```python
from build123d import *

# Parameters (mm, degrees)
SKETCH1_W                   = 3.2
SKETCH1_H                   = 10.1
BOSS_EXTRUDE1_DEPTH         = 3
SENSOR_MOUNTING_HOLES_REACH = 85.637
SKETCH2_R                   = 1.6
SKETCH2_R_2                 = 1.5
SKETCH2_R_3                 = 3.1
SKETCH2_W                   = 9.5
SKETCH2_H                   = 8
SKETCH2_W_2                 = 29.5
SKETCH2_H_2                 = 8.4
SKETCH2_W_3                 = 11.5
SKETCH2_H_3                 = 13
SKETCH2_W_4                 = 12
SKETCH2_H_4                 = 11


with BuildPart() as part:
    # Sketch1 → Boss-Extrude1 (new body)
    with BuildSketch(Plane.XY):
        with BuildLine():
            Line((-58.19, 60), (58.19, 60))
            Line((58.19, 60), (58.19, 3))
            Line((58.19, 3), (11.618950039, 3))
            ThreePointArc((11.618950039, 3), (0, 12), (-11.618950039, 3))
            Line((-11.618950039, 3), (-58.19, 3))
            Line((-58.19, 3), (-58.19, 60))
        make_face()
        with Locations((-52.69, 15)):
            Rectangle(SKETCH1_W, SKETCH1_H, mode=Mode.SUBTRACT)
        with Locations((-52.69, 48)):
            Rectangle(SKETCH1_W, SKETCH1_H, mode=Mode.SUBTRACT)
        with Locations((52.69, 15)):
            Rectangle(SKETCH1_W, SKETCH1_H, mode=Mode.SUBTRACT)
        with Locations((52.69, 48)):
            Rectangle(SKETCH1_W, SKETCH1_H, mode=Mode.SUBTRACT)
    extrude(amount=-BOSS_EXTRUDE1_DEPTH)

    # Sketch2 (on Front Plane) → sensor mounting holes (cut, up to next)
    with BuildSketch(Plane.XY, mode=Mode.PRIVATE) as sensor_mounting_holes_sk1:
        with Locations((-18, 44)):
            Circle(SKETCH2_R)
    sensor_mounting_holes_tool1 = extrude(sensor_mounting_holes_sk1.sketch, amount=-SENSOR_MOUNTING_HOLES_REACH, mode=Mode.PRIVATE) & part.part
    # Sketch2 (on Front Plane) → sensor mounting holes (cut, up to next)
    with BuildSketch(Plane.XY, mode=Mode.PRIVATE) as sensor_mounting_holes_sk2:
        with Locations((18, 44)):
            Circle(SKETCH2_R)
    sensor_mounting_holes_tool2 = extrude(sensor_mounting_holes_sk2.sketch, amount=-SENSOR_MOUNTING_HOLES_REACH, mode=Mode.PRIVATE) & part.part
    # Sketch2 (on Front Plane) → sensor mounting holes (cut, up to next)
    with BuildSketch(Plane.XY, mode=Mode.PRIVATE) as sensor_mounting_holes_sk3:
        with Locations((-22.118932188, 29.071067812)):
            Circle(SKETCH2_R_2)
    sensor_mounting_holes_tool3 = extrude(sensor_mounting_holes_sk3.sketch, amount=-SENSOR_MOUNTING_HOLES_REACH, mode=Mode.PRIVATE) & part.part
    # Sketch2 (on Front Plane) → sensor mounting holes (cut, up to next)
    with BuildSketch(Plane.XY, mode=Mode.PRIVATE) as sensor_mounting_holes_sk4:
        with Locations((-36.261067812, 29.071067812)):
            Circle(SKETCH2_R_2)
    sensor_mounting_holes_tool4 = extrude(sensor_mounting_holes_sk4.sketch, amount=-SENSOR_MOUNTING_HOLES_REACH, mode=Mode.PRIVATE) & part.part
    # Sketch2 (on Front Plane) → sensor mounting holes (cut, up to next)
    with BuildSketch(Plane.XY, mode=Mode.PRIVATE) as sensor_mounting_holes_sk5:
        with Locations((-36.261067812, 14.928932188)):
            Circle(SKETCH2_R_2)
    sensor_mounting_holes_tool5 = extrude(sensor_mounting_holes_sk5.sketch, amount=-SENSOR_MOUNTING_HOLES_REACH, mode=Mode.PRIVATE) & part.part
    # Sketch2 (on Front Plane) → sensor mounting holes (cut, up to next)
    with BuildSketch(Plane.XY, mode=Mode.PRIVATE) as sensor_mounting_holes_sk6:
        with Locations((-22.118932188, 14.928932188)):
            Circle(SKETCH2_R_2)
    sensor_mounting_holes_tool6 = extrude(sensor_mounting_holes_sk6.sketch, amount=-SENSOR_MOUNTING_HOLES_REACH, mode=Mode.PRIVATE) & part.part
    # Sketch2 (on Front Plane) → sensor mounting holes (cut, up to next)
    with BuildSketch(Plane.XY, mode=Mode.PRIVATE) as sensor_mounting_holes_sk7:
        with Locations((-29.19, 22)):
            Circle(SKETCH2_R_2)
    sensor_mounting_holes_tool7 = extrude(sensor_mounting_holes_sk7.sketch, amount=-SENSOR_MOUNTING_HOLES_REACH, mode=Mode.PRIVATE) & part.part
    # Sketch2 (on Front Plane) → sensor mounting holes (cut, up to next)
    with BuildSketch(Plane.XY, mode=Mode.PRIVATE) as sensor_mounting_holes_sk8:
        with Locations((30.240588995, 13.245945843)):
            Circle(SKETCH2_R_3)
    sensor_mounting_holes_tool8 = extrude(sensor_mounting_holes_sk8.sketch, amount=-SENSOR_MOUNTING_HOLES_REACH, mode=Mode.PRIVATE) & part.part
    # Sketch2 (on Front Plane) → sensor mounting holes (cut, up to next)
    with BuildSketch(Plane.XY, mode=Mode.PRIVATE) as sensor_mounting_holes_sk9:
        with Locations((16.44, 27)):
            Rectangle(SKETCH2_W, SKETCH2_H)
    sensor_mounting_holes_tool9 = extrude(sensor_mounting_holes_sk9.sketch, amount=-SENSOR_MOUNTING_HOLES_REACH, mode=Mode.PRIVATE) & part.part
    # Sketch2 (on Front Plane) → sensor mounting holes (cut, up to next)
    with BuildSketch(Plane.XY, mode=Mode.PRIVATE) as sensor_mounting_holes_sk10:
        with Locations((0, 44)):
            Rectangle(SKETCH2_W_2, SKETCH2_H_2)
    sensor_mounting_holes_tool10 = extrude(sensor_mounting_holes_sk10.sketch, amount=-SENSOR_MOUNTING_HOLES_REACH, mode=Mode.PRIVATE) & part.part
    # Sketch2 (on Front Plane) → sensor mounting holes (cut, up to next)
    with BuildSketch(Plane.XY, mode=Mode.PRIVATE) as sensor_mounting_holes_sk11:
        Polygon((24.912246381, 42.955051143), (29.112246381, 42.955051143), (29.112246381, 51.455051143), (32.612246381, 51.455051143), (32.612246381, 25.155051143), (29.112246381, 25.155051143), (29.112246381, 34.655051143), (24.912246381, 34.655051143), align=None)
    sensor_mounting_holes_tool11 = extrude(sensor_mounting_holes_sk11.sketch, amount=-SENSOR_MOUNTING_HOLES_REACH, mode=Mode.PRIVATE) & part.part
    # Sketch2 (on Front Plane) → sensor mounting holes (cut, up to next)
    with BuildSketch(Plane.XY, mode=Mode.PRIVATE) as sensor_mounting_holes_sk12:
        with Locations((41.090588995, 19.745945843)):
            Rectangle(SKETCH2_W_3, SKETCH2_H_3)
    sensor_mounting_holes_tool12 = extrude(sensor_mounting_holes_sk12.sketch, amount=-SENSOR_MOUNTING_HOLES_REACH, mode=Mode.PRIVATE) & part.part
    # Sketch2 (on Front Plane) → sensor mounting holes (cut, up to next)
    with BuildSketch(Plane.XY, mode=Mode.PRIVATE) as sensor_mounting_holes_sk13:
        with Locations((40.362246381, 49.88070744)):
            Rectangle(SKETCH2_W_4, SKETCH2_H_4)
    sensor_mounting_holes_tool13 = extrude(sensor_mounting_holes_sk13.sketch, amount=-SENSOR_MOUNTING_HOLES_REACH, mode=Mode.PRIVATE) & part.part
    add(sensor_mounting_holes_tool1.solids().sort_by_distance((-18, 44, 0))[0], mode=Mode.SUBTRACT)
    add(sensor_mounting_holes_tool2.solids().sort_by_distance((18, 44, 0))[0], mode=Mode.SUBTRACT)
    add(sensor_mounting_holes_tool3.solids().sort_by_distance((-22.118932, 29.071068, 0))[0], mode=Mode.SUBTRACT)
    add(sensor_mounting_holes_tool4.solids().sort_by_distance((-36.261068, 29.071068, 0))[0], mode=Mode.SUBTRACT)
    add(sensor_mounting_holes_tool5.solids().sort_by_distance((-36.261068, 14.928932, 0))[0], mode=Mode.SUBTRACT)
    add(sensor_mounting_holes_tool6.solids().sort_by_distance((-22.118932, 14.928932, 0))[0], mode=Mode.SUBTRACT)
    add(sensor_mounting_holes_tool7.solids().sort_by_distance((-29.19, 22, 0))[0], mode=Mode.SUBTRACT)
    add(sensor_mounting_holes_tool8.solids().sort_by_distance((30.240589, 13.245946, 0))[0], mode=Mode.SUBTRACT)
    add(sensor_mounting_holes_tool9.solids().sort_by_distance((16.44, 27, 0))[0], mode=Mode.SUBTRACT)
    add(sensor_mounting_holes_tool10.solids().sort_by_distance((0, 44, 0))[0], mode=Mode.SUBTRACT)
    add(sensor_mounting_holes_tool11.solids().sort_by_distance((29.804717, 38.442393, 0))[0], mode=Mode.SUBTRACT)
    add(sensor_mounting_holes_tool12.solids().sort_by_distance((41.090589, 19.745946, 0))[0], mode=Mode.SUBTRACT)
    add(sensor_mounting_holes_tool13.solids().sort_by_distance((40.362246, 49.880707, 0))[0], mode=Mode.SUBTRACT)


solid = part.part
```
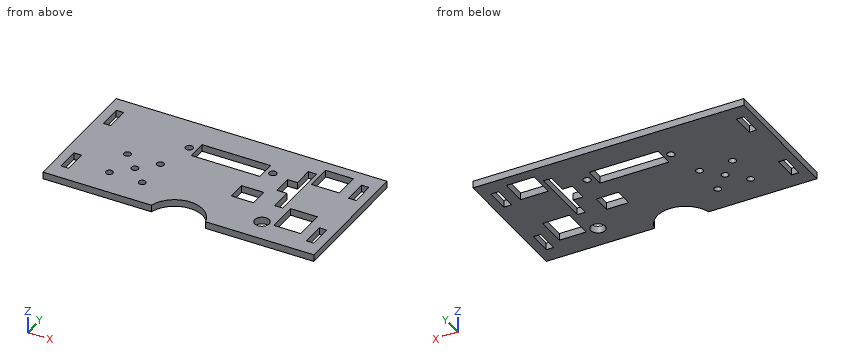
CAD build for the part. Positions are in the model's coordinates, mm. Round coordinates to 2 decimals unless told otherwise and drop trailing zeros. Write each loop counter-clockwise with the first axis right and the second up, starting at its lowest first coordinate (ties: lowest second). Pieces come first, ordered by that corner, then holes. Notation, with made-up numbers: (49.5, 39) -> (77.5, 39) arc R25 ccw to (77.5, 60) -> close; hole circle Ø10 at (24.5, -31.75). An arc over 180 degrees is marked (long way). Answer in a Markdown table with one row per item. Add a question column.
Item 1: Drill centre lines: line 1 (Y direction, x = 43, z = -0.8); line 2 (X direction, y = 41.5, z = -1.9); line 3 (X direction, y = 52, z = -1.6). Where is each one in solid material? Low to high. Write a range as from..to.
Item 2: Saw through at B-B, the plane y = 6. Write the cut outline in (x, z), then the cut area to 3 significant figures.
Item 3: Saw through at C-C, the plane z = -1.85. Count the separate pieces of the cut face and the enclosed holes in it, then the cut area to 3 significant figures.
Item 4: Saw through at A-A, the plane x = 26. Write the cut outline in (y, z).
Item 5: Drop flat-ended pins along their axis: pin 1 Ø2.5 at (x, y) = (-18, 44) entering from +Z; pin 2 Ø1 at (x, y) = (-30, 29) entering from +Z. Give the stop position or say it passes through.
Findings below:
| question | item | result |
|---|---|---|
| 1 | line 1 | y = 3..13.25, 26.25..44.38, 55.38..60 |
| 1 | line 2 | x = -58.19..-14.75, 14.75..24.91, 32.61..58.19 |
| 1 | line 3 | x = -58.19..-54.29, -51.09..34.36, 46.36..51.09, 54.29..58.19 |
| 2 | outline | (-58.19, -3) -> (-10.39, -3) -> (-10.39, 0) -> (-58.19, 0) -> close; (10.39, -3) -> (58.19, -3) -> (58.19, 0) -> (10.39, 0) -> close |
| 2 | area | 287 mm^2 |
| 3 | separate pieces | 1 |
| 3 | enclosed holes | 17 |
| 3 | area | 5,540 mm^2 |
| 4 | outline | (3, -3) -> (34.66, -3) -> (34.66, 0) -> (3, 0) -> close; (42.96, -3) -> (60, -3) -> (60, 0) -> (42.96, 0) -> close |
| 5 | pin 1 | passes through |
| 5 | pin 2 | stops at z = 0 |
